```python
from build123d import *

# Parameters (mm, degrees)
BOSS_EXTRUDE1_DEPTH = 1.524


with BuildPart() as part:
    # Sketch1 → Boss-Extrude1 (new body)
    with BuildSketch(Plane.XY):
        with BuildLine():
            Line((66.817686168, -14.869164569), (59.056150877, -13.876858964))
            Line((59.056150877, -13.876858964), (59.247042617, -12.382986483))
            Line((59.247042617, -12.382986483), (67.194822679, -13.398359477))
            ThreePointArc((67.194822679, -13.398359477), (67.70899541, -13.26788211), (67.995751093, -12.821598434))
            ThreePointArc((67.995751093, -12.821598434), (64.227291304, -9.497799736), (61.607555958, -5.209919876))
            ThreePointArc((61.607555958, -5.209919876), (61.375328576, -6.683073901), (60.554429435, -7.928159013))
            Line((60.554429435, -7.928159013), (57.70805725, -7.403828432))
            ThreePointArc((57.70805725, -7.403828432), (50.857364323, -5.31551987), (45.193330731, -0.93239887))
            ThreePointArc((45.193330731, -0.93239887), (46.74856309, -5.980463476), (46.532138914, -11.258234267))
            ThreePointArc((46.532138914, -11.258234267), (45.814421681, -11.988335606), (44.917143983, -12.481345467))
            ThreePointArc((44.917143983, -12.481345467), (38.532037538, -13.275274102), (32.219333695, -14.520134408))
            ThreePointArc((32.219333695, -14.520134408), (26.075931145, -13.405705196), (19.832270887, -13.398359477))
            ThreePointArc((19.832270887, -13.398359477), (22.636275156, -14.465946733), (24.725407976, -16.619480236))
            ThreePointArc((24.725407976, -16.619480236), (19.193818209, -18.629561925), (13.804325827, -20.994363314))
            ThreePointArc((13.804325827, -20.994363314), (11.961969019, -21.092468706), (10.589989147, -19.858947525))
            ThreePointArc((10.589989147, -19.858947525), (8.692873036, -16.140740523), (6.604648633, -12.52640356))
            ThreePointArc((6.604648633, -12.52640356), (8.591060293, -11.950308262), (10.589989147, -12.481345467))
            ThreePointArc((10.589989147, -12.481345467), (6.604648633, -8.173624539), (1.539487899, -5.209919876))
            ThreePointArc((1.539487899, -5.209919876), (-4.115983201, 1.303955497), (-10.439102907, 7.171926434))
            ThreePointArc((-10.439102907, 7.171926434), (-8.653197321, 7.552707081), (-6.867291735, 7.171926434))
            ThreePointArc((-6.867291735, 7.171926434), (-13.248231641, 12.071035928), (-20.796462113, 14.853460169))
            ThreePointArc((-20.796462113, 14.853460169), (-31.29237864, 21.067135925), (-42.647396117, 25.521078925))
            ThreePointArc((-42.647396117, 25.521078925), (-56.186845853, 26.702409902), (-69.371487811, 30.000509128))
            ThreePointArc((-69.371487811, 30.000509128), (-65.415318989, 26.726735017), (-60.436877471, 25.468168876))
            ThreePointArc((-60.436877471, 25.468168876), (-57.284615578, 25.003207948), (-54.152019191, 24.420298363))
            ThreePointArc((-54.152019191, 24.420298363), (-48.766215804, 22.329910268), (-44.346090572, 18.609817064))
            ThreePointArc((-44.346090572, 18.609817064), (-44.75848849, 20.197264615), (-44.346090572, 21.784712166))
            ThreePointArc((-44.346090572, 21.784712166), (-35.698486655, 18.358779729), (-27.477516693, 14.007490327))
            ThreePointArc((-27.477516693, 14.007490327), (-24.652349792, 11.020731115), (-23.207012071, 7.171926434))
            ThreePointArc((-23.207012071, 7.171926434), (-21.929330632, 8.763840822), (-19.890640696, 8.865843888))
            ThreePointArc((-19.890640696, 8.865843888), (-14.26749676, 4.199817582), (-9.066352318, -0.93239887))
            ThreePointArc((-9.066352318, -0.93239887), (-6.212207546, -5.345518339), (-5.336411329, -10.527674919))
            ThreePointArc((-5.336411329, -10.527674919), (-4.676038807, -8.910060646), (-3.250173943, -7.900269978))
            ThreePointArc((-3.250173943, -7.900269978), (2.428109507, -16.545845472), (7.012996253, -25.817721879))
            ThreePointArc((7.012996253, -25.817721879), (9.928518411, -28.520179408), (13.883000235, -28.113215463))
            ThreePointArc((13.883000235, -28.113215463), (14.506734037, -27.753899557), (15.133981782, -27.400753634))
            ThreePointArc((15.133981782, -27.400753634), (19.438401061, -26.804711741), (23.74282034, -27.400753634))
            ThreePointArc((23.74282034, -27.400753634), (23.721132898, -25.36083225), (22.275997143, -23.920925222))
            ThreePointArc((22.275997143, -23.920925222), (30.525936774, -21.012373591), (39.064631831, -19.111883331))
            ThreePointArc((39.064631831, -19.111883331), (45.641469135, -19.389960489), (51.636059466, -22.1097036))
            ThreePointArc((51.636059466, -22.1097036), (51.007316283, -20.144641068), (51.693543332, -18.19890697))
            ThreePointArc((51.693543332, -18.19890697), (55.664100075, -18.365490547), (59.619700642, -18.74797596))
            ThreePointArc((59.619700642, -18.74797596), (63.927856855, -18.638412611), (67.326700796, -15.988870395))
            ThreePointArc((67.326700796, -15.988870395), (67.384238378, -15.287162887), (66.817686168, -14.869164569))
        make_face()
    extrude(amount=BOSS_EXTRUDE1_DEPTH)


solid = part.part
```
Part model, mm, in its own coordinate system. A direction names the side the tool comes from. Give positions to 0.01 mm unless a question says otherwise; leave off trailing zeros. Order: outer loops, then holes, each group sorted by start corner. A loop starts at its lowest first (then second) coordinate and runs counter-clockwise, first axis right, second up. Notation, with made-up numbers: M 4,-6.75 L 11,-6.75 A15 cw 11,-0.75 Z; hole C 3,-10.5 d6. An arc over 180 degrees is marked long. Use a Markdown table: item, result. Add a question column.
(1) Saw through at A-A, the plane y = 12. Give the cut face in (x, z).
(2) 3-axis set-ups, long thin cutter, end or side, ignore diameter. For faces 4 (the face through (19.27, -18.6, 0.75)), 5 (the face through (50.947, -5.362, 0.751)), 6 (the face through (-14.343, 4.268, 0.751)): which of +Z, -Z, +X, -X, +Y, -Y reach the whole face in a straight line?
(3) Probe line 1 along X through (y, z) = (-9.5, 0.9); line 2 along X through (y, z) = (19.5, 1.3); line 3 along X through (y, z) = (20, 0.3). List the from-to ranges inside material, lowest first. Write a range as [from, to].
(4) Saw through at B-B, the plane x = 27. Give the cut face in (y, z), and give its area (3 significant figures).
(5) Mould opens along X. For faces 1 (the face through (22.6, -14.44, 0.75)), 2 (the face through (-56, 26.67, 0.75)), 3 (the face through (9.87, -28.5, 0.75)) say: +X half, -X half, draft (parallel to the pull), parting line (faces both ways), or undercut.
Answer key:
| question | item | result |
|---|---|---|
| 1 | outline | M -25.35,0 L -13.12,0 L -13.12,1.52 L -25.35,1.52 Z |
| 2 | face 4 | +Z, -Z |
| 2 | face 5 | +Z, -Z, +Y |
| 2 | face 6 | +Z, -Z, -Y |
| 3 | line 1 | [-5.34, -5.05], [-2.08, 8.1], [46.8, 64.23] |
| 3 | line 2 | [-45.16, -44.68], [-38.29, -28.26] |
| 3 | line 3 | [-45.67, -44.75], [-39.5, -29.19] |
| 4 | outline | M -22.12,0 L -13.5,0 L -13.5,1.52 L -22.12,1.52 Z |
| 4 | area | 13.1 mm^2 |
| 5 | face 1 | undercut |
| 5 | face 2 | +X half |
| 5 | face 3 | parting line |
